Source: CAD feature listing. Evaluate the final solid. Frame: model axes, mm. Face numbers are marked on the shaded views. A direction names the side the tool comes from. Coordinates: 2 decimals unless noted, no trailing zeros. Write each loop counter-clockwise with the first axis right and the second up, starting at its lowest first coordinate (ties: lowest second). Pieces come first, ordered by that corner, then holes. Notation, with made-up numbers: (-3, -33) - (19, -33) arc R10 cw to (19, -26) - close; hole circle Ø10 at (25.25, 63). An arc over 180 degrees is marked (long way). One line per question, with ' | ' between items. Start each with the question number.
Q1. Access query for the marked faces 1 and 2. Directions: +Z, -Z, +X, -X, +Y, -Y. A direction counts if a zero-diameter tool reaches every point of the face in a straight line with its end or side. Return the directions, or none.
Q2. Cut plane B-B, the plane x = 1. Return loops of the section in (y, z).
Q3. Draft query along X for the marked faces 3, 4 and 5. Return one class per face: +X half, -X half, draft (parallel to the pull), parting line (faces both ways), or undercut.
Q4. Line query: line 1 (X direction, y = 0, z = -10.75); line 2 (X direction, y = -2, z = -14.5). Output: solid intervals per line, ascending.
Q5. Cut plane D-D, the plane x = 3.75. Return loops of the section in (y, z).
Q6. Contact query for a flat-ended pin moving along its axis: P1, Ø2.5, axis at x = 0, y = 0, coming from the +Z side. Output: stop coordinate, or through.
Q7. Cut plane A-A, the plane z = -4.5. Return loops of the section in (x, y).
Autodesk Fusion 360 part; units mm, degrees
sketch "Sketch1" plane through (0, 0, 0) normal (0, 0, 1) x (1, 0, 0)
  line L0 (1.651, -1.651) -> (-1.651, -1.651)
  line L1 (-1.651, -1.651) -> (-1.651, 1.651)
  line L2 (-1.651, 1.651) -> (1.651, 1.651)
  line L3 (1.651, 1.651) -> (1.651, -1.651)
  line L4 (1.651, -1.651) -> (-1.651, 1.651) construction
  line L5 (-1.651, -1.651) -> (1.651, 1.651) construction
  line L6 (4.318, -4.318) -> (-4.318, -4.318)
  line L7 (-4.318, -4.318) -> (-4.318, 4.318)
  line L8 (-4.318, 4.318) -> (4.318, 4.318)
  line L9 (4.318, 4.318) -> (4.318, -4.318)
  line L10 (4.318, -4.318) -> (-4.318, 4.318) construction
  line L11 (-4.318, -4.318) -> (4.318, 4.318) construction
  dimension "d1" = 3.302
extrude "Extrude1" add sketch "Sketch1" against normal blind 12
sketch "Sketch2" plane through (0, 0, -12) normal (0, 0, -1) x (1, 0, 0)
  line L0 (1.651, -1.651) -> (-1.651, -1.651)
  line L1 (-1.651, -1.651) -> (-1.651, 1.651)
  line L2 (-1.651, 1.651) -> (1.651, 1.651)
  line L3 (1.651, 1.651) -> (1.651, -1.651)
  line L4 (-4.318, -4.318) -> (4.318, -4.318)
  line L5 (4.318, -4.318) -> (4.318, 4.318)
  line L6 (4.318, 4.318) -> (-4.318, 4.318)
  line L7 (-4.318, 4.318) -> (-4.318, -4.318)
  line L8 (-4.318, 4.318) -> (4.318, 4.318)
  line L9 (4.318, 4.318) -> (4.318, -4.318)
  line L10 (4.318, -4.318) -> (-4.318, -4.318)
  line L11 (-4.318, -4.318) -> (-4.318, 4.318)
extrude "Extrude2" add sketch "Sketch2" along normal blind 3 contours L0 L1 L2 L3 | L4 L5 L6 L7 L8 L9 L10 L11
fillet "Fillet1" radius 1 4 edges at (-4.318, 4.318, -7.5) (4.318, 4.318, -7.5) (4.318, -4.318, -7.5) (-4.318, -4.318, -7.5)
fillet "Fillet2" radius 1 8 edges at (-4.0251, -4.0251, -15) (-4.318, 0, -15) (-4.0251, 4.0251, -15) (0, 4.318, -15) (4.0251, 4.0251, -15) (4.318, 0, -15) (4.0251, -4.0251, -15) (0, -4.318, -15)
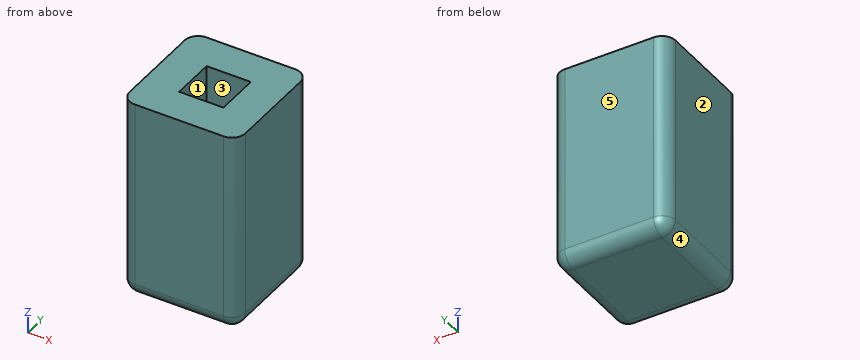
Reply:
1) face 1: +Z | face 2: +Z, -Z, -X, +Y, -Y
2) outline: (-4.32, -14) arc R1 ccw to (-3.32, -15) - (3.32, -15) arc R1 ccw to (4.32, -14) - (4.32, 0) - (1.65, 0) - (1.65, -12) - (-1.65, -12) - (-1.65, 0) - (-4.32, 0) - close
3) face 3: undercut | face 4: -X half | face 5: draft
4) line 1: x = -4.32 to -1.65, 1.65 to 4.32 | line 2: x = -4.18 to 4.18
5) outline: (-4.22, -14) arc R0.9 ccw to (-3.32, -14.9) - (3.32, -14.9) arc R0.9 ccw to (4.22, -14) - (4.22, 0) - (-4.22, 0) - close
6) P1: stops at z = -12
7) outline: (-4.32, -3.32) arc R1 ccw to (-3.32, -4.32) - (3.32, -4.32) arc R1 ccw to (4.32, -3.32) - (4.32, 3.32) arc R1 ccw to (3.32, 4.32) - (-3.32, 4.32) arc R1 ccw to (-4.32, 3.32) - close; hole (-1.65, -1.65) - (1.65, -1.65) - (1.65, 1.65) - (-1.65, 1.65) - close
